Geometry check sheet. Reference: drawing and pictorial views, mm from the part's lowest x, y, z. A direction names the side the tool comes from. Give positions to 0.01 mm unless a question says otherwise; leave off trailing zeros. Order: outer loops, then holes, each group sorted by start corner. A loop starts at its lowest first (then second) coordinate and runs counter-clockwise, first axis right, second up.
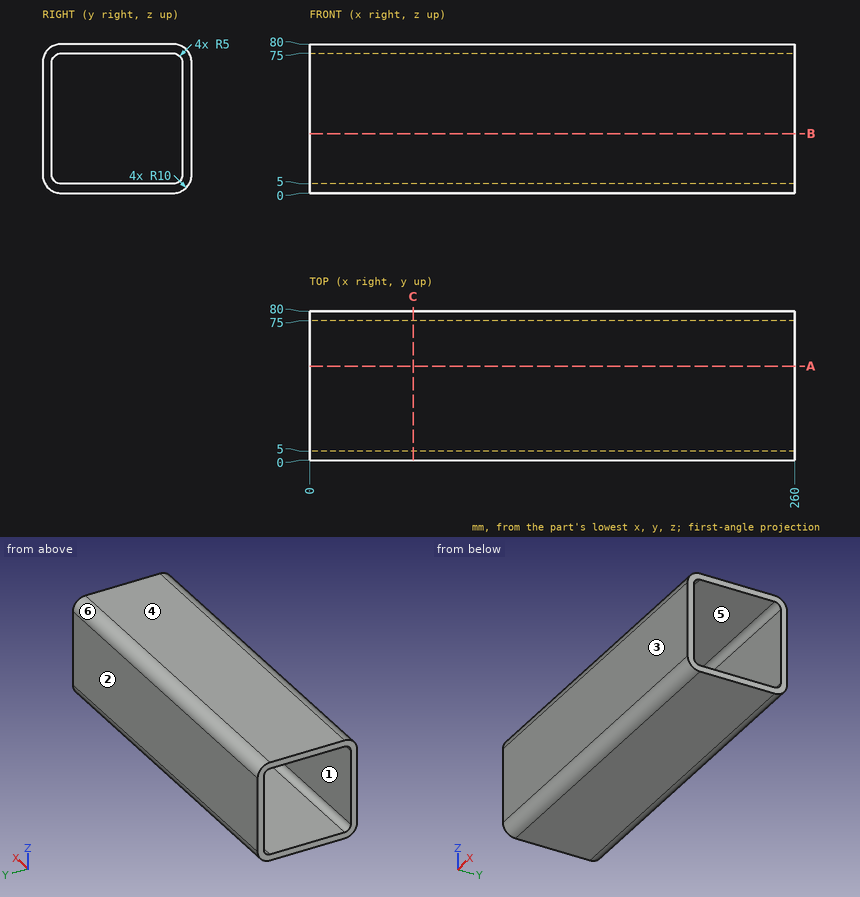
(1) Release check for a two-part mould opening along Y. For the marked faces 1, 2, 3 and 4 record: released by +Y, released by -Y, zero draft, split by the parting line, or undercut.
Response values:
face 1: undercut
face 2: released by +Y
face 3: released by -Y
face 4: zero draft
(2) Set-up check for the marked faces 5 and 6: record each of +Z, -Z, +X, -X, +Y, -Y from which the full face is reachable in a straight line by a thin tool's end or side.
Response values:
face 5: +X, -X
face 6: +Z, +X, -X, +Y
(3) Cross-section at C-C on x = 55.5. Enter the section's corners in (y, z), then the cut area to 3 significant figures.
Response values:
outline: (0, 10) arc R10 ccw to (10, 0) - (70, 0) arc R10 ccw to (80, 10) - (80, 70) arc R10 ccw to (70, 80) - (10, 80) arc R10 ccw to (0, 70) - close; hole (5, 10) arc R5 ccw to (10, 5) - (70, 5) arc R5 ccw to (75, 10) - (75, 70) arc R5 ccw to (70, 75) - (10, 75) arc R5 ccw to (5, 70) - close
area: 1,440 mm2
(4) Material ranges on L1, parallel to Z at x = 12.5, y = 57; L2, parallel to Y at x = 123, z = 7, recorded low to high.
Response values:
L1: z = 0 to 5, 75 to 80
L2: y = 0.46 to 6, 74 to 79.54
(5) Cross-section at A-A on y = 50.5. Enter the section's corners in (x, z).
Response values:
outline: (0, 0) - (260, 0) - (260, 5) - (0, 5) - close; (0, 75) - (260, 75) - (260, 80) - (0, 80) - close
